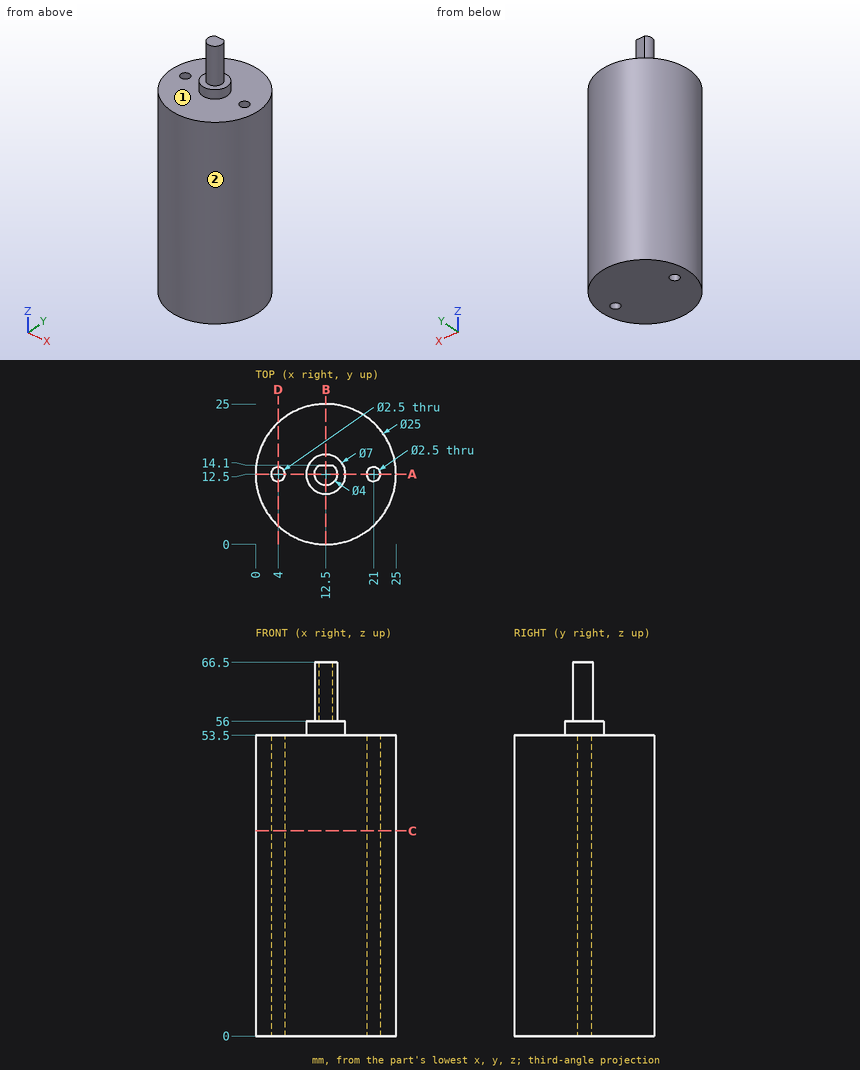
Check sheet for the drawn part. Datum: minimum x, y, z corner. Units: mm. A direction names the side the tool comes from. Round coordinates to 2 decimals unless told otherwise and drop trailing zeros. Order: outer loops, then holes, each group sorted by start corner. A loop starts at its lowest first (then second) coordinate and runs counter-clockwise, first axis right, second up. Notation, with made-up numbers: (0.25, -3) -> (42.25, -3) arc R11 cw to (42.25, 18) -> close; hole circle Ø3 at (-1.5, -17.5). An arc over 180 degrees is marked (long way). Put each result on its own line as item: value.
1) Set-up check for the marked faces 1 and 2: record each of +Z, -Z, +X, -X, +Y, -Y from which the full face is reachable in a straight line by a thin tool's end or side.
Final values:
face 1: +Z
face 2: +Z, -Z
2) Section check C-C (z = 36.5). Record the cut outline in (x, y), then the cut area to 3 significant figures.
Final values:
outline: circle Ø25 at (12.5, 12.5); hole circle Ø2.5 at (4, 12.5); hole circle Ø2.5 at (21, 12.5)
area: 481 mm^2
3) Depth check by flat-ended pin: pin 1 (1.5 mm diameter, centred on x = 22.5, z = 50.5, fed in from +Y); pin 2 (2.5 mm diameter, centred on x = 12, z = 60, fed in from +Y); pin 3 (4 mm diameter, centred on x = 7.5, y = 10.5, fed in from +Z). Enter the tip coordinate at first touch or a pass-through.
Final values:
pin 1: stops at y = 20.91
pin 2: stops at y = 14.1
pin 3: stops at z = 56
4) Section check D-D (x = 4). Record the cut outline in (y, z).
Final values:
outline: (3.33, 0) -> (11.25, 0) -> (11.25, 53.5) -> (3.33, 53.5) -> close; (13.75, 0) -> (21.67, 0) -> (21.67, 53.5) -> (13.75, 53.5) -> close
5) Section check A-A (y = 12.5). Record the cut outline in (x, z), then the cut area to 3 significant figures.
Final values:
outline: (0, 0) -> (2.75, 0) -> (2.75, 53.5) -> (0, 53.5) -> close; (5.25, 0) -> (19.75, 0) -> (19.75, 53.5) -> (16, 53.5) -> (16, 56) -> (14.5, 56) -> (14.5, 66.5) -> (10.5, 66.5) -> (10.5, 56) -> (9, 56) -> (9, 53.5) -> (5.25, 53.5) -> close; (22.25, 0) -> (25, 0) -> (25, 53.5) -> (22.25, 53.5) -> close
area: 1,130 mm^2
6) Material ranges on line 1 (Z direction, x = 8, y = 11); line 2 (Z direction, x = 14, y = 9.75); line 3 (Y direction, x = 4, z = 15), recorded low to high.
Final values:
line 1: z = 0 to 53.5
line 2: z = 0 to 56
line 3: y = 3.33 to 11.25, 13.75 to 21.67
7) Section check B-B (x = 12.5). Record the cut outline in (y, z), then the cut area to 3 significant figures.
Final values:
outline: (0, 0) -> (25, 0) -> (25, 53.5) -> (16, 53.5) -> (16, 56) -> (14.1, 56) -> (14.1, 66.5) -> (10.5, 66.5) -> (10.5, 56) -> (9, 56) -> (9, 53.5) -> (0, 53.5) -> close
area: 1,390 mm^2
